```python
from build123d import *

# Parameters (mm, degrees)
SKETCH2_R          = 3.048
CUT_EXTRUDE1_DEPTH = 2.54


# Read off the part's stored shape, not the designer's step: Revolve1
with BuildPart() as part:
    # Revolve1 outline → Revolve1 (revolve)
    with BuildSketch(Plane(origin=(-9.292485091, 0, 0), x_dir=(1, 0, 0), z_dir=(0, 0, 1))):
        Polygon((0, -15.377840902), (0, -24.394840902), (1.27, -24.394840902), (1.27, -22.108840902), (3.048, -22.108840902), (3.048, -20.838840902), (1.6764, -20.838840902), (1.6764, -15.377840902), align=None)
    revolve(axis=Axis((-9.292485091, 0, 0), (0, 1, 0)))

    # Sketch2 → Cut-Extrude1 (cut)
    with BuildSketch(Plane(origin=(0, -20.838840902, 0), x_dir=(1, 0, 0), z_dir=(0, 1, 0))):
        with Locations((-9.292485091, 0)):
            Circle(SKETCH2_R)
        Polygon((-9.292485091, 2.286), (-7.312751018, 1.143), (-7.312751018, -1.143), (-9.292485091, -2.286), (-11.272219164, -1.143), (-11.272219164, 1.143), align=None, mode=Mode.SUBTRACT)
    extrude(amount=-CUT_EXTRUDE1_DEPTH, mode=Mode.SUBTRACT)


solid = part.part
```
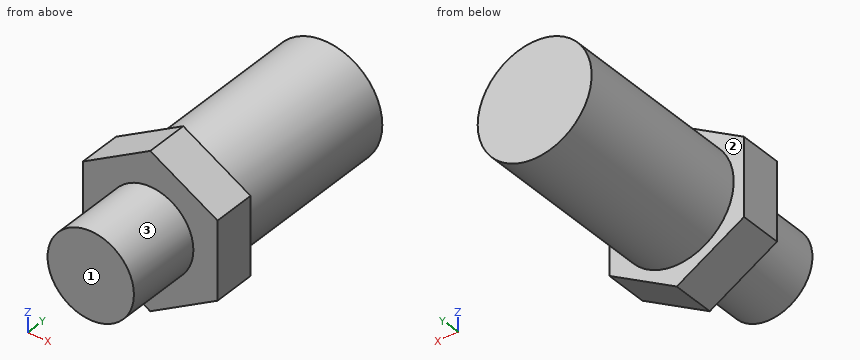
Verification items for the finished model (mm, model axes). Face numbers are marked on the shaded views. A direction names the side the tool comes from. Round coordinates to 2 decimals unless told otherwise and drop trailing zeros. Write each loop counter-clockwise with the first axis right and the second up, starting at its lowest first coordinate (ties: lowest second). Pieces come first, ordered by that corner, then holes.
1. Scan lines: L1, parallel to Y at x = -10.85, z = 0.95; L2, parallel to Y at x = -8, z = 0.9; L3, parallel to X at y = -22.25, z = 0.05. Record each from-to range of solid material in increasing order.
2. Section check A-A on z = 0. Enter the section's corners in (x, y).
3. Gauge pin test, flat ends, axial feed: P1, Ø1, axis at x = -10, y = -17, coming from the +Z side; P2, Ø1.5, axis at y = -17, z = 1, coming from the -X side. Record the tip position at first contact, or that the pin passes through.
4. Access from +Z, -Z, +X, -X, +Y, -Y to the whole of each face (thin tool, end or side, straight path). Record for the marked faces 1, 2 and 3.
5. Section check B-B on x = -9.6. Enter the section's corners in (y, z), plus the area to 3 significant figures.
6. Section check D-D on z = -1.45. Enter the section's corners in (x, y).
7. Section check C-C on y = -22. Enter the section's corners in (x, z), plus the area to 3 significant figures.
Answer:
1. L1: y = -22.11 to -20.84
1. L2: y = -22.11 to -15.38
1. L3: x = -10.56 to -8.02
2. outline: (-11.27, -22.11) - (-10.56, -22.11) - (-10.56, -24.39) - (-8.02, -24.39) - (-8.02, -22.11) - (-7.31, -22.11) - (-7.31, -20.84) - (-7.62, -20.84) - (-7.62, -15.38) - (-10.97, -15.38) - (-10.97, -20.84) - (-11.27, -20.84) - close
3. P1: stops at z = 1.66
3. P2: stops at x = -10.95
4. face 1: +Z, -Z, +X, -X, -Y
4. face 2: +Y
4. face 3: -Y
5. outline: (-24.39, -1.23) - (-22.11, -1.23) - (-22.11, -2.11) - (-20.84, -2.11) - (-20.84, -1.65) - (-15.38, -1.65) - (-15.38, 1.65) - (-20.84, 1.65) - (-20.84, 2.11) - (-22.11, 2.11) - (-22.11, 1.23) - (-24.39, 1.23) - close
5. area: 29.0 mm2
6. outline: (-10.74, -22.11) - (-7.84, -22.11) - (-7.84, -20.84) - (-8.45, -20.84) - (-8.45, -15.38) - (-10.13, -15.38) - (-10.13, -20.84) - (-10.74, -20.84) - close
7. outline: (-11.27, -1.14) - (-9.29, -2.29) - (-7.31, -1.14) - (-7.31, 1.14) - (-9.29, 2.29) - (-11.27, 1.14) - close
7. area: 13.6 mm2
